```python
from build123d import *

# Parameters (mm, degrees)
EXTRUDE1_DEPTH             = 40
SKETCH2_R                  = 1.2
EXTRUDE2_DEPTH             = 4.8
SKETCH_R                   = 2.1
SKETCH_R_2                 = 1.2
EXTRUDE4_DEPTH             = 2.3
CHAMFER1_SIZE              = 0.2
LPATTERN1_COUNT            = 3
LPATTERN1_PITCH            = 15
CHAMFER1_OF_LPATTERN1_SIZE = 0.2


with BuildPart() as part:
    # Sketch1 → Extrude1 (new body)
    with BuildSketch(Plane.XY):
        with BuildLine():
            Line((-3.3, -2.4), (3.3, -2.4))
            Line((3.3, -2.4), (3.5, -2.2))
            Line((3.5, -2.2), (3.5, 0.106274607))
            ThreePointArc((3.5, 0.106274607), (3.091294745, 0.282570681), (2.840065792, 0.65))
            Line((2.840065792, 0.65), (2.340065792, 0.65))
            Line((2.340065792, 0.65), (2.340065792, 1.15))
            Line((2.340065792, 1.15), (2.840065792, 1.15))
            ThreePointArc((2.840065792, 1.15), (3.091294745, 1.517429319), (3.5, 1.693725393))
            Line((3.5, 1.693725393), (3.5, 2.2))
            Line((3.5, 2.2), (3.3, 2.4))
            Line((3.3, 2.4), (-3.3, 2.4))
            Line((-3.3, 2.4), (-3.5, 2.2))
            Line((-3.5, 2.2), (-3.5, 1.693725393))
            ThreePointArc((-3.5, 1.693725393), (-3.091294745, 1.517429319), (-2.840065792, 1.15))
            Line((-2.840065792, 1.15), (-2.340065792, 1.15))
            Line((-2.340065792, 1.15), (-2.340065792, 0.65))
            Line((-2.340065792, 0.65), (-2.840065792, 0.65))
            ThreePointArc((-2.840065792, 0.65), (-3.091294745, 0.282570681), (-3.5, 0.106274607))
            Line((-3.5, 0.106274607), (-3.5, -2.2))
            Line((-3.5, -2.2), (-3.3, -2.4))
        make_face()
    extrude(amount=EXTRUDE1_DEPTH)

    # Sketch2 → Extrude2 (cut)
    with BuildSketch(Plane(origin=(0, 2.4, 0), x_dir=(1, 0, 0), z_dir=(0, 1, 0))):
        with Locations((0, -5)):
            Circle(SKETCH2_R)
    extrude2 = extrude(amount=-EXTRUDE2_DEPTH, mode=Mode.SUBTRACT)

    # Sketch → Extrude4 (cut)
    with BuildSketch(Plane(origin=(0, 2.4, 0), x_dir=(1, 0, 0), z_dir=(0, 1, 0))):
        with Locations((0, -5)):
            Circle(SKETCH_R)
        with Locations((0, -5)):
            Circle(SKETCH_R_2, mode=Mode.SUBTRACT)
    extrude4 = extrude(amount=-EXTRUDE4_DEPTH, mode=Mode.SUBTRACT)

    # Chamfer1
    chamfer1_edges = [part.edges().sort_by_distance(p)[0] for p in [
        (-1.2, -2.4, 5),
        (-2.1, 2.4, 5),
    ]]
    chamfer(chamfer1_edges, length=CHAMFER1_SIZE)

    # LPattern1: Extrude2, Extrude4 ×3
    with Locations(*[(0, 0, i * LPATTERN1_PITCH) for i in range(1, LPATTERN1_COUNT)]):
        add(extrude2, mode=Mode.SUBTRACT)
        add(extrude4, mode=Mode.SUBTRACT)

    # Chamfer1 of LPattern1
    chamfer1_of_lpattern1_edges = [part.edges().sort_by_distance(p)[0] for p in [
        (-1.2, -2.4, 20),
        (-2.1, 2.4, 20),
        (-1.2, -2.4, 35),
        (-2.1, 2.4, 35),
    ]]
    chamfer(chamfer1_of_lpattern1_edges, length=CHAMFER1_OF_LPATTERN1_SIZE)


solid = part.part
```
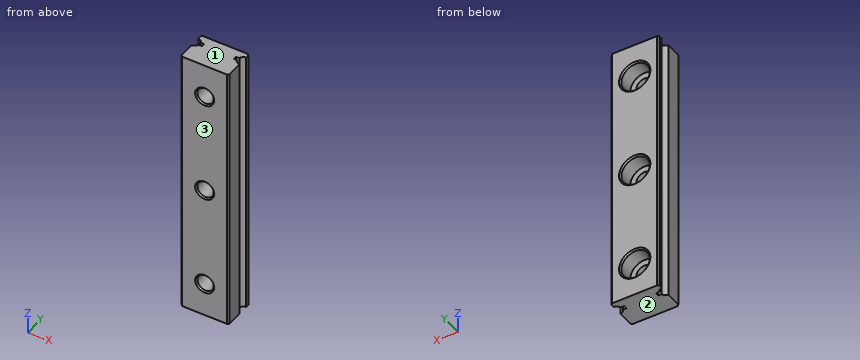
For this review, take the finished solid that the model builds, in its own axes (mm). Face numbers are marked on the shaded views. Coordinates: 2 decimals unless noted, no trailing zeros. Write each loop counter-clockwise with the first axis right and the second up, starting at its lowest first coordinate (ties: lowest second). Pieces come first, ordered by that corner, then holes. Notation, with made-up numbers: (52, 74.5) - (94, 74.5) arc R22 cw to (94, 81.5) - close; hole circle Ø3 at (-33, 80). An arc over 180 degrees is marked (long way). Put each result on its own line as item: value.
1. Mouldability with a two-part tool opening along Z and no side actions: class the marked faces 1, 2 and 3 as released by +Z, released by -Z, zero draft, split by the parting line, or undercut.
Values found:
face 1: released by +Z
face 2: released by -Z
face 3: zero draft
2. Add section B-B, the plane y = -0.65. Give the boundary of the cut face in (x, z).
Values found:
outline: (-3.5, 0) - (3.5, 0) - (3.5, 40) - (-3.5, 40) - close; hole circle Ø2.4 at (0, 5); hole circle Ø2.4 at (0, 20); hole circle Ø2.4 at (0, 35)
3. Add section D-D, the plane x = 0. Count the separate pieces of the cut face and the enclosed holes in it, then the cut area to 3 significant figures.
Values found:
separate pieces: 4
enclosed holes: 0
area: 145 mm²
4. For pin 1 (3 mm diameter, centred on x = 0, z = 5, fed in from +Y); pin 2 (4 mm diameter, centred on x = 0, z = 35, fed in from -Y); pin 3 (2 mm diameter, centred on x = 0, z = 20, fed in from -Y), all flat-tipped, find the tip position at first contact; note any pin that passes through.
Values found:
pin 1: y = 0.1
pin 2: y = -2.4
pin 3: through
5. Add section C-C, the plane z = 27.5. Give the boundary of the cut face in (x, y), then the cut area to 3 significant figures.
Values found:
outline: (-3.5, -2.2) - (-3.3, -2.4) - (3.3, -2.4) - (3.5, -2.2) - (3.5, 0.11) arc R0.8 cw to (2.84, 0.65) - (2.34, 0.65) - (2.34, 1.15) - (2.84, 1.15) arc R0.8 cw to (3.5, 1.69) - (3.5, 2.2) - (3.3, 2.4) - (-3.3, 2.4) - (-3.5, 2.2) - (-3.5, 1.69) arc R0.8 cw to (-2.84, 1.15) - (-2.34, 1.15) - (-2.34, 0.65) - (-2.84, 0.65) arc R0.8 cw to (-3.5, 0.11) - close
area: 31.4 mm²
6. Wall thickness on probe 1 along Z at (x, y) = (0, 0.9); probe 2 along Z at (x, y) = (0, -1.25); probe 3 along X at (y, z) = (-1.15, 20): over which ranges is each line inside the solid? List them lowest first.
Values found:
probe 1: 0 to 2.9, 7.1 to 17.9, 22.1 to 32.9, 37.1 to 40
probe 2: 0 to 3.8, 6.2 to 18.8, 21.2 to 33.8, 36.2 to 40
probe 3: -3.5 to -1.2, 1.2 to 3.5
